from build123d import *

# Parameters (mm, degrees)
SKETCH1_W           = 44.6
SKETCH1_H           = 18.8
BOSS_EXTRUDE1_DEPTH = 2.5
SKETCH2_W           = 12.7
SKETCH2_H           = 7.62
BOSS_EXTRUDE2_DEPTH = 20
FILLET1_R           = 2
FILLET2_R           = 0.5


with BuildPart() as part:
    # Sketch1 → Boss-Extrude1 (new body)
    with BuildSketch(Plane(origin=(0, 0, 0), x_dir=(1, 0, 0), z_dir=(0, 1, 0))):
        with Locations((0, 6.65)):
            Rectangle(SKETCH1_W, SKETCH1_H)
    extrude(amount=-BOSS_EXTRUDE1_DEPTH)

    # Sketch2 → Boss-Extrude2 (add)
    with BuildSketch(Plane(origin=(0, 0, 0), x_dir=(1, 0, 0), z_dir=(0, 1, 0))):
        with Locations((0, 1.81)):
            Rectangle(SKETCH2_W, SKETCH2_H)
    extrude(amount=-BOSS_EXTRUDE2_DEPTH)

    # Fillet1
    fillet1_edges = [part.edges().sort_by_distance(p)[0] for p in [
        (6.35, -20, -1.81),
        (0, -20, 2),
        (-6.35, -20, -1.81),
        (0, -20, -5.62),
    ]]
    fillet(fillet1_edges, radius=FILLET1_R)

    # Fillet2
    fillet2_edges = [part.edges().sort_by_distance(p)[0] for p in [
        (6.35, -2.5, -1.81),
        (0, -2.5, 2),
        (-6.35, -2.5, -1.81),
        (0, -2.5, -5.62),
    ]]
    fillet(fillet2_edges, radius=FILLET2_R)


solid = part.part
Read the model definition and answer for the solid it produces. Units are mm, in the model's axes. A direction names the side the tool comes from. Coordinates: 2 decimals unless noted, no trailing zeros. Loops run counter-clockwise (first coordinate to the right, second up) from the corner with the lowest first, then second, coordinate; pieces in that order, holes last. Notation, with made-up numbers: (80, 42.25) -> (125, 42.25) arc R8 cw to (125, 51.25) -> close; hole circle Ø3 at (-39.75, 84). An arc over 180 degrees is marked (long way). Answer in a Markdown table with one row per item.
Item 1: For a pull along Z with two mould halves and no side action, classify faces 6 (the flat face through (0, -10, 2)), 7 (the flat face through (0, -20, -2)), 8 (the flat face through (0, -1, -16.05)) as released by +Z, released by -Z, zero draft, split by the parting line, or undercut.
Returned:
| item | result |
|---|---|
| face 6 | released by +Z |
| face 7 | zero draft |
| face 8 | released by -Z |
Item 2: A cutting plane is placed at B-B on z = 0.5. Determine the outline of the cut face in (x, y), plus the area to 3 significant figures.
Returned:
| item | result |
|---|---|
| outline | (-22.3, -2.5) -> (-6.85, -2.5) arc R0.5 cw to (-6.35, -3) -> (-6.35, -18) arc R2 ccw to (-4.85, -19.94) -> (4.85, -19.94) arc R2 ccw to (6.35, -18) -> (6.35, -3) arc R0.5 cw to (6.85, -2.5) -> (22.3, -2.5) -> (22.3, 0) -> (-22.3, 0) -> close |
| area | 332 mm^2 |
Item 3: For faces 1 (the flat face through (0, 0, -7)), 2 (the flat face through (-6.35, -10, -2)), 3 (the flat face through (6.35, -10, -2)), 4 (the cylindrical face through (0.09, -19.4, 1.43)), 5 (the flat face through (0, -10, -5.62)), determine the directions among +Z, -Z, +X, -X, +Y, -Y from which every point of the face is accessible in a straight line to the end or side of a thin tool.
Returned:
| item | result |
|---|---|
| face 1 | +Z, -Z, +X, -X, +Y |
| face 2 | +Z, -Z, -X, -Y |
| face 3 | +Z, -Z, +X, -Y |
| face 4 | +Z, +X, -X, -Y |
| face 5 | -Z, +X, -X, -Y |
Item 4: Each of these flat-tipped pins is pushed along its axis until it touches: P1, Ø2.5, axis at y = -8, z = -2.5, coming from the +X side; P2, Ø10, axis at y = -14, z = -4, coming from the -X side; P3, Ø1, axis at x = -13, z = -11, coming from the -Y side. Where does it stop, or does it pass through?
Returned:
| item | result |
|---|---|
| P1 | stops at x = 6.35 |
| P2 | stops at x = -6.35 |
| P3 | stops at y = -2.5 |
Item 5: A cutting plane is placed at C-C on y = -4.25. Determine the outline of the cut face in (x, z), plus the area to 3 significant figures.
Returned:
| item | result |
|---|---|
| outline | (-6.35, -5.62) -> (6.35, -5.62) -> (6.35, 2) -> (-6.35, 2) -> close |
| area | 96.8 mm^2 |
Item 6: A cutting plane is placed at D-D on z = -13.25. Determine the outline of the cut face in (x, y).
Returned:
| item | result |
|---|---|
| outline | (-22.3, -2.5) -> (22.3, -2.5) -> (22.3, 0) -> (-22.3, 0) -> close |
Item 7: Straight lines are drawn through the part: line 1 along Z through (x, y) = (0.5, -9.25); line 2 along X through (y, z) = (-3.25, -0.25); line 3 along Y through (x, z) = (8.5, -7). For each, find the intervals that lie inside material, in ascending order. Write a range as [from, to].
Returned:
| item | result |
|---|---|
| line 1 | z = [-5.62, 2] |
| line 2 | x = [-6.35, 6.35] |
| line 3 | y = [-2.5, 0] |
Item 8: A cutting plane is placed at A-A on x = 5.5. Determine the outline of the cut face in (y, z), plus the area to 3 significant figures.
Returned:
| item | result |
|---|---|
| outline | (-19.64, -4.77) arc R2 ccw to (-18, -5.62) -> (-3, -5.62) arc R0.5 cw to (-2.5, -6.12) -> (-2.5, -16.05) -> (0, -16.05) -> (0, 2.75) -> (-2.5, 2.75) -> (-2.5, 2.5) arc R0.5 cw to (-3, 2) -> (-18, 2) arc R2 ccw to (-19.64, 1.15) -> close |
| area | 177 mm^2 |
